```python
from build123d import *

# Parameters (mm, degrees)
MOTOR_SHAFT_DEPTH  = 13
SKETCH4_R          = 1.5
STRING_HOLES_DEPTH = 17.5
FILLET1_R          = 2


with BuildPart() as part:
    # Sketch2 → Revolve1 (revolve)
    with BuildSketch(Plane.XY, mode=Mode.PRIVATE) as revolve1_sk:
        Polygon((15, 14), (15, 19), (17, 19), (17, 0), (-17, 0), (-17, 19), (-15, 19), (-15, 14), (-4, 7), (4, 7), align=None)
    revolve(revolve1_sk.sketch.rotate(Axis((0, 0, 0), (1, 0, 0)), 90), axis=Axis((0, 0, 0), (1, 0, 0)))

    # Sketch3 → motor shaft (cut)
    with BuildSketch(Plane.ZY.offset(17)):
        with BuildLine():
            Line((2.9, 1.574801575), (2.9, -1.574801575))
            ThreePointArc((2.9, -1.574801575), (-3.3, 0), (2.9, 1.574801575))
        make_face()
    extrude(amount=-MOTOR_SHAFT_DEPTH, mode=Mode.SUBTRACT)

    # Sketch4 → string holes (cut, symmetric)
    with BuildSketch(Plane.XY):
        Circle(SKETCH4_R)
    extrude(amount=STRING_HOLES_DEPTH, both=True, mode=Mode.SUBTRACT)

    # Fillet1
    fillet1_edges = [part.edges().sort_by_distance(p)[0] for p in [
        (15, 0, -14),
        (-15, 0, -14),
    ]]
    fillet(fillet1_edges, radius=FILLET1_R)


solid = part.part
```
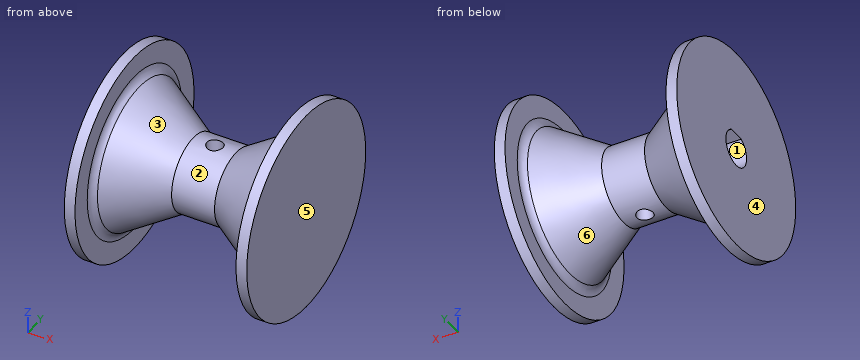
Check sheet for the modelled part. Datum: model origin and axes. Units: mm. Face numbers are marked on the shaded views. A direction names the side the tool comes from. Coordinates: 2 decimals unless noted, no trailing zeros. Write each loop counter-clockwise with the first axis right and the second up, starting at its lowest first coordinate (ties: lowest second). Pieces come first, ordered by that corner, then holes. Notation, with made-up numbers: (54, 89) - (61, 89) arc R12 cw to (61, 95) - close; hole circle Ø11 at (36, -30.5). An arc over 180 degrees is marked (long way). One line per question, with ' | ' between items.
Item 1: Sectioned sample at B-B on z = 0. Record the boundary of the cut face in (x, y).
Determined:
outline: (-17, -19) - (-15, -19) - (-15, -15.1) arc R2 cw to (-14.07, -13.41) - (-4, -7) - (4, -7) - (14.07, -13.41) arc R2 cw to (15, -15.1) - (15, -19) - (17, -19) - (17, 19) - (15, 19) - (15, 15.1) arc R2 cw to (14.07, 13.41) - (4, 7) - (-4, 7) - (-14.07, 13.41) arc R2 cw to (-15, 15.1) - (-15, 19) - (-17, 19) - (-17, 3.3) - (-4, 3.3) - (-4, -3.3) - (-17, -3.3) - close; hole circle Ø3 at (0, 0)
Item 2: Mould release check, pull along X, two halves, no side actions. Record for the marked faces 1, 2, 3 and 4: pulls with the +X half, pulls with the -X half, needs draft (parallel to the pull), parting line crosses it, or undercut.
Determined:
face 1: needs draft | face 2: undercut | face 3: undercut | face 4: pulls with the -X half
Item 3: Sectioned sample at D-D on x = -12. Record the boundary of the cut face in (y, z), plus the area to 3 significant figures.
Determined:
outline: circle Ø24.18 at (0, 0); hole (-1.57, 2.9) arc R3.3 ccw (long way) to (1.57, 2.9) - close | area: 426 mm2
Item 4: Thickness scan on line 1 (Y direction, x = 0, z = 0.25); line 2 (X direction, y = 0, z = 1.25); line 3 (X direction, y = -12, z = 6). Record the ranges inside material, lowest first. Write a range as [from, to].
Determined:
line 1: y = [-7, -1.5], [1.5, 7] | line 2: x = [-4, -1.5], [1.5, 17] | line 3: x = [-17, -14.08], [14.08, 17]
Item 5: Sectioned sample at C-C on x = 0. Record the boundary of the cut face in (y, z).
Determined:
outline: (-1.5, -6.84) - (-1.5, 6.84) arc R7 ccw to start; (1.5, -6.84) arc R7 ccw to (1.5, 6.84) - close
Item 6: Sectioned sample at A-A on y = 0. Record the boundary of the cut face in (x, z), plus the area to 3 significant figures.
Determined:
outline: (-17, -19) - (-15, -19) - (-15, -15.1) arc R2 cw to (-14.07, -13.41) - (-4, -7) - (-1.5, -7) - (-1.5, 7) - (-4, 7) - (-14.07, 13.41) arc R2 cw to (-15, 15.1) - (-15, 19) - (-17, 19) - (-17, 2.9) - (-4, 2.9) - (-4, -3.3) - (-17, -3.3) - close; (1.5, -7) - (4, -7) - (14.07, -13.41) arc R2 cw to (15, -15.1) - (15, -19) - (17, -19) - (17, 19) - (15, 19) - (15, 15.1) arc R2 cw to (14.07, 13.41) - (4, 7) - (1.5, 7) - close | area: 604 mm2
Item 7: Access from +Z, -Z, +X, -X, +Y, -Y to the whole of each face (thin tool, end or side, straight path). Record for the marked faces 5 and 6.
Determined:
face 5: +Z, -Z, +X, +Y, -Y | face 6: none
Item 8: Gauge pin test, flat ends, axial feed: P1, Ø4, axis at x = 2.5, z = -10, coming from the -Y side; P2, Ø12, axis at x = 13.5, z = -0.5, coming from the +Y side; P3, Ø1.9, axis at y = -0.5, z = 1, coming from the -X side; P4, Ø2, axis at x = -9.5, z = -6, coming from the +Y side. Record the tip position at first contact, or that the pin passes through.
Determined:
P1: passes through | P2: stops at y = 19 | P3: stops at x = -4 | P4: stops at y = 9.59
